from build123d import *

# Parameters (mm, degrees)
SKETCH6_W                = 9.525
SKETCH6_H                = 38.1
BOSS_EXTRUDE2_DEPTH      = 263.525
SKETCH7_R                = 4.7625
CUT_EXTRUDE2_DEPTH       = 367.423749955
FILLET2_R                = 3.175
CIRPATTERN2_COUNT        = 3
FILLET2_OF_CIRPATTERN2_R = 3.175
CHAMFER5_SIZE            = 0.635
CHAMFER6_SIZE            = 1.27


with BuildPart() as part:
    # Sketch5 → Base-Revolve (revolve)
    with BuildSketch(Plane.XY, mode=Mode.PRIVATE) as base_revolve_sk:
        Polygon((12.7, 173.99), (6.35, 173.99), (6.35, 179.07), (12.7, 179.07), (12.7, 196.596), (6.35, 196.596), (6.35, 201.676), (12.7, 201.676), (12.7, 254), (0, 254), (0, 0), (12.7, 0), align=None)
    revolve(base_revolve_sk.sketch.rotate(Axis((0, 112.385522388, 0), (0, -1, 0)), 90), axis=Axis((0, 112.385522388, 0), (0, -1, 0)))

    # Sketch6 → Boss-Extrude2 (add)
    with BuildSketch(Plane.XY):
        with Locations((0, 19.05)):
            Rectangle(SKETCH6_W, SKETCH6_H)
    boss_extrude2 = extrude(amount=BOSS_EXTRUDE2_DEPTH)

    # Sketch7 → Cut-Extrude2 (cut, through all)
    with BuildSketch(Plane(origin=(4.7625, 0, 0), x_dir=(0, 0, -1), z_dir=(1, 0, 0))):
        with Locations(Location((-257.175, 31.75, 0), (0, 0, 90))):
            Circle(SKETCH7_R)
    cut_extrude2 = extrude(amount=-CUT_EXTRUDE2_DEPTH, mode=Mode.SUBTRACT)

    # Fillet2
    fillet2_edges = [part.edges().sort_by_distance(p)[0] for p in [
        (-4.7625, 19.05, 11.773215098),
        (4.7625, 19.05, 11.773215098),
    ]]
    fillet(fillet2_edges, radius=FILLET2_R)

    # CirPattern2: Boss-Extrude2, Cut-Extrude2 ×3 about axis
    cirpattern2_axis = Axis((0, 0, 0), (0, 1, 0))
    add([boss_extrude2.rotate(cirpattern2_axis, i * 360 / CIRPATTERN2_COUNT) for i in range(1, CIRPATTERN2_COUNT)])
    add([cut_extrude2.rotate(cirpattern2_axis, i * 360 / CIRPATTERN2_COUNT) for i in range(1, CIRPATTERN2_COUNT)], mode=Mode.SUBTRACT)

    # Fillet2 of CirPattern2
    fillet2_of_cirpattern2_edges = [part.edges().sort_by_distance(p)[0] for p in [
        (12.577153359, 19.05, -1.762161564),
        (7.814653359, 19.05, -10.011053535),
        (-7.814653359, 19.05, -10.011053535),
        (-12.577153359, 19.05, -1.762161564),
    ]]
    fillet(fillet2_of_cirpattern2_edges, radius=FILLET2_OF_CIRPATTERN2_R)

    # Chamfer5
    chamfer5_edges = [part.edges().sort_by_distance(p)[0] for p in [
        (0, 179.07, -12.7),
        (0, 196.596, -12.7),
        (0, 201.676, -12.7),
        (0, 173.99, -12.7),
    ]]
    chamfer(chamfer5_edges, length=CHAMFER5_SIZE)

    # Chamfer6
    chamfer6_edges = [part.edges().sort_by_distance(p)[0] for p in [
        (0, 254, -12.7),
    ]]
    chamfer(chamfer6_edges, length=CHAMFER6_SIZE)


solid = part.part
Input: part model. Units: mm. Frame: model coordinates. A direction names the side the tool comes from. Give positions to 0.01 mm unless a question says otherwise; leave off trailing zeros. Loops run counter-clockwise (first coordinate to the right, second up) from the corner with the lowest first, then second, coordinate; pieces in that order, holes last. Notation, with made-up numbers: (68.25, -14.5) -> (110.25, -14.5) arc R33 cw to (110.25, 14.5) -> close; hole circle Ø5 at (8.5, 6). An arc over 180 degrees is marked (long way). Answer as a JSON object with one key per item and string values. Group by question number.
Item 1: Reachability of faces 5 (the flat face through (5, 201.676, -5)), 6 (the flat face through (-4.762, 19, 137)), 7 (the cylindrical face through (7.7, 227.9, -10.1)) from +Z, -Z, +X, -X, +Y, -Y: full face, straight path, thin tool, end or side. Return the list, or none.
Item 2: Line query: probe 1 along Z at (x, y) = (-0.75, 31.75) (1 decimal); probe 2 along Z at (x, y) = (-1.5, 31.75) (1 decimal); probe 3 along X at (y, z) = (101.5, -5). Output: solid intervals per line, ascending.
Item 3: Cut plane A-A, the plane z = -83.5. Return the cut outline in (x, y).
Item 4: Cut plane C-C, the plane z = 100.5. Return the cut outline in (x, y), and give its area (3 significant figures).
Item 5: Pull-direction query (Z, two-part tool) for faces 1 (the cylindrical face through (3.86, 176.57, -5.04)), 2 (the cylindrical face through (-225.54, 28.24, -130.14)), 3 (the flat face through (0, 38.1, 135)), 4 (the flat face through (-116.17, 18.78, -72.57)); classes: released by +Z, released by -Z, zero draft, split by the parting line, or undercut.
Item 6: Pin query (flat end, axial travel): P1, Ø11, axis at y = 31.75, z = 257.175, coming from the +X side; P2, Ø6.5, axis at x = 0, z = 122, coming from the +Y side; P3, Ø6, axis at y = 151.5, z = 10, coming from the +X side. Return the tip coordinate at first contact, or that it passes through.
Item 7: Cut plane B-B, the plane y = 117.5. Return the cut outline in (x, z), and give its area (3 significant figures).
Item 8: Cut plane D-D, the plane x = -76. Return the cut outline in (y, z).
Checks:
{
 "1": {"face 5": "none", "face 6": "+Z, -X, +Y, -Y", "face 7": "+Y"},
 "2": {"probe 1": "z = -12.7 to 252.4, 261.9 to 263.5", "probe 2": "z = -12.6 to 252.4, 261.9 to 263.5", "probe 3": "x = -11.67 to 11.67"},
 "3": {"outline": "(-154.15, 0) -> (-135.1, 0) -> (-135.1, 38.1) -> (-154.15, 38.1) -> close; (135.1, 0) -> (154.15, 0) -> (154.15, 38.1) -> (135.1, 38.1) -> close"},
 "4": {"outline": "(-4.76, 0) -> (4.76, 0) -> (4.76, 38.1) -> (-4.76, 38.1) -> close", "area": "363 mm²"},
 "5": {"face 1": "split by the parting line", "face 2": "undercut", "face 3": "zero draft", "face 4": "released by -Z"},
 "6": {"P1": "stops at x = 4.76", "P2": "stops at y = 38.1", "P3": "stops at x = 10.6"},
 "7": {"outline": "circle Ø25.4 at (0, 0)", "area": "507 mm²"},
 "8": {"outline": "(0, -49.38) -> (38.1, -49.38) -> (38.1, -38.38) -> (0, -38.38) -> close"}
}
